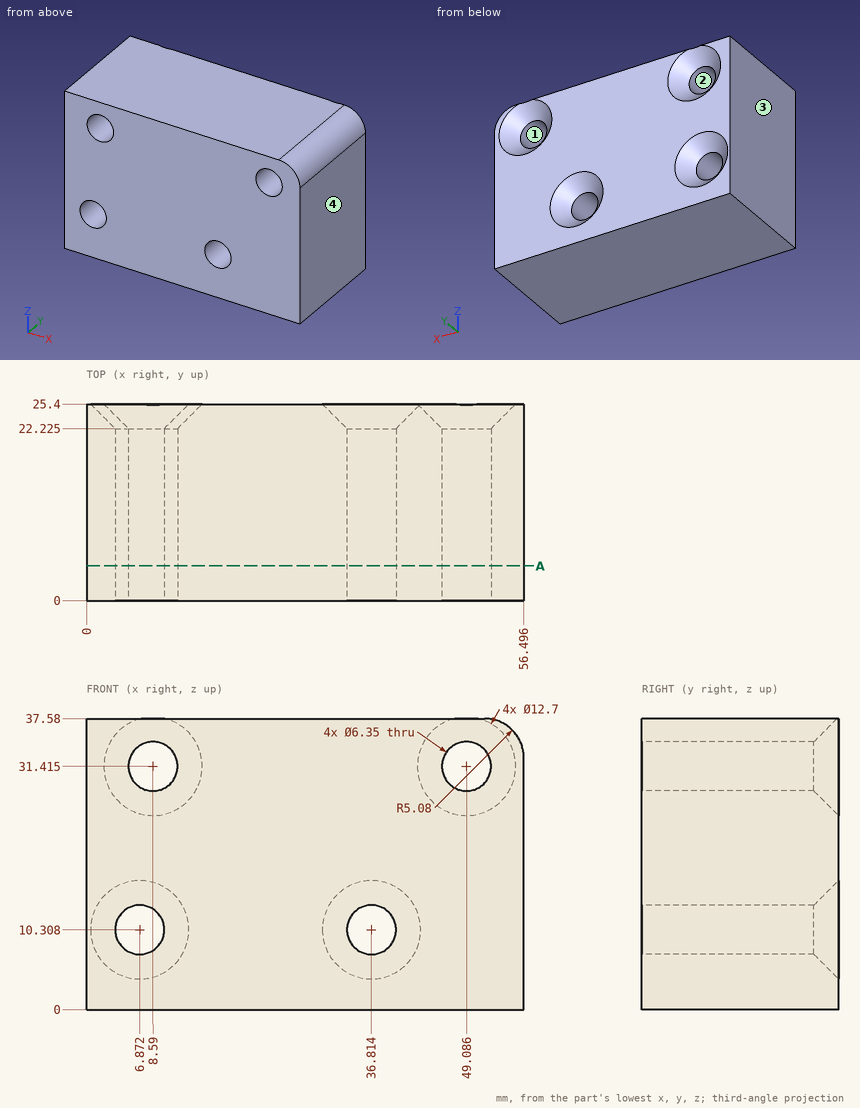
Can you work these out from the drawing? Everything is in mm from the part's minimum corner. Give positions to 0.01 mm unless a question says otherwise; leave off trailing zeros. Answer in a Markdown table with one row per item. Add a question column.
Item 1: For pin 1 Ø4 at (x, z) = (9.5, 13) entering from -Y; pin 2 Ø10 at (x, z) = (36.81, 10.31) entering from +Y (1 decimal), each with a flat end and sliding along its axis, tell me the tip position at first contact or that it passes through.
Item 2: Imagine slicing it at A-A, the plane y = 4.5. State how many separate pieces and enclosed holes the cut face has, plus the area to 3 significant figures.
Item 3: Please list where these lines run through material, in increasing order: L1, parallel to X at y = 19, z = 31.5; L2, parallel to Z at x = 38, y = 1.5; L3, parallel to X at y = 17, z = 33 (1 decimal).
Item 4: We'd pull the mould along X, two halves only. Please class the marked faces 1, 2, 3 and 4: released by +X, released by -X, zero draft, split by the parting line, or undercut.
Evaluation:
| question | item | result |
|---|---|---|
| 1 | pin 1 | stops at y = 0 |
| 1 | pin 2 | stops at y = 24.1 |
| 2 | separate pieces | 1 |
| 2 | enclosed holes | 4 |
| 2 | area | 1,990 mm² |
| 3 | L1 | x = 0 to 5.42, 11.76 to 45.91, 52.26 to 56.5 |
| 3 | L2 | z = 0 to 7.36, 13.25 to 37.58 |
| 3 | L3 | x = 0 to 5.8, 11.3 to 46.3, 51.8 to 56.5 |
| 4 | face 1 | undercut |
| 4 | face 2 | undercut |
| 4 | face 3 | released by -X |
| 4 | face 4 | released by +X |
